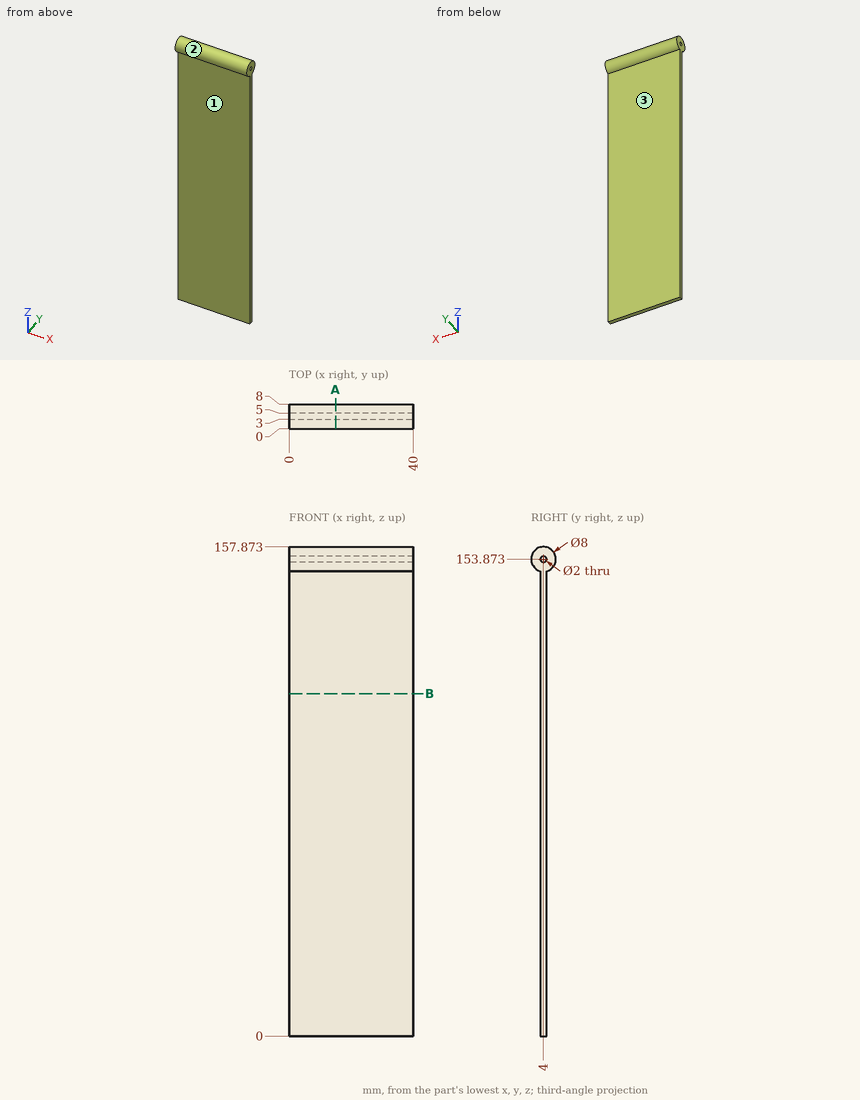
Source: three-view drawing plus pictorial views. Frame: mm from the lowest corner of the part. A direction names the side the tool comes from. Round coordinates to 2 decimals unless told otherwise and drop trailing zeros. Loops run counter-clockwise (first coordinate to the right, second up) from the corner with the lowest first, then second, coordinate; pieces in that order, holes last. Notation, with made-up numbers: M 70,32 L 74,32 A21 cw 74,45 Z; hole C 69.5,61.25 d3. An arc over 180 degrees is marked long. Put each result on its own line as item: value.
(1) First-contact query: pin 1 (3 mm diameter, centred on x = 16.5, z = 117.5, fed in from -Y); pin 2 (2 mm diameter, centred on x = 23.5, y = 1, fed in from -Z); pin 3 (1 mm diameter, centred on y = 4, z = 82.5, fed in from -X); pin 4 (12 mm diameter, centred on x = 11.5, z = 92, fed in from +Y). Flat tips, straight axial feed; report the tip coordinate or a pass-through.
Solutions:
pin 1: y = 3
pin 2: z = 150.41
pin 3: x = 0
pin 4: y = 5
(2) Section B-B, the plane z = 110.5. Return loops of the section in (x, y).
Solutions:
outline: M 0,3 L 40,3 L 40,5 L 0,5 Z
(3) Ray query, line 1 (Z direction, x = 9.5, y = 3.75); line 2 (Y direction, x = 25.5, z = 84); line 3 (Z direction, x = 13, y = 5.5). Return the intervals inside material, ascending. Write a range as [from, to].
Solutions:
line 1: [0, 152.9], [154.84, 157.87]
line 2: [3, 5]
line 3: [150.16, 157.58]
(4) Access query for the marked faces 1, 2 and 3. Directions: +Z, -Z, +X, -X, +Y, -Y. A direction counts if a zero-diameter tool reaches every point of the face in a straight line with its end or side. Return the directions, or none.
Solutions:
face 1: -Z, +X, -X, -Y
face 2: +X, -X
face 3: -Z, +X, -X, +Y
(5) Section A-A, the plane x = 15. Return loops of the section in (y, z), and give its area (3 significant figures).
Solutions:
outline: M 3,0 L 5,0 L 5,150 A4 ccw long 3,150 Z; hole C 4,153.87 d2
area: 347 mm²
